The model under review builds one solid part; all positions refer to its coordinate system, in mm. Face numbers are marked on the shaded views. A direction names the side the tool comes from. Round coordinates to 2 decimals unless told otherwise and drop trailing zeros. Loops run counter-clockwise (first coordinate to the right, second up) from the corner with the lowest first, then second, coordinate; pieces in that order, holes last. Notation, with made-up numbers: (-13, -18.5) - (-9, -18.5) arc R24 cw to (-9, 19.5) - close; hole circle Ø11 at (-27, -18.5). An arc over 180 degrees is marked (long way). Answer as CSV lines item,"result".
Autodesk Fusion 360 part; units mm, degrees
sketch "Sketch1" plane through (0, 0, 0) normal (0, 0, 1) x (1, 0, 0)
  line L0 (67.5, 27.5) -> (-67.5, 27.5)
  line L1 (-67.5, 27.5) -> (-67.5, -27.5)
  line L2 (-67.5, -27.5) -> (67.5, -27.5)
  line L3 (67.5, -27.5) -> (67.5, 27.5)
  line L4 (67.5, 27.5) -> (-67.5, -27.5) construction
  line L5 (-67.5, 27.5) -> (67.5, -27.5) construction
  dimension "d1" = 55
  dimension "d2" = 135
extrude "Extrude1" add sketch "Sketch1" along normal blind 6 makes body 1
sketch "Sketch3" plane through (0, 0, 0) normal (0, 0, -1) x (-1, 0, 0)
  line L0 (-67.5, 27.5) -> (-67.5, -27.5)
  line L1 (-67.5, -27.5) -> (67.5, -27.5)
  line L2 (67.5, -27.5) -> (67.5, 27.5)
  line L3 (67.5, 27.5) -> (-67.5, 27.5)
  line L4 (-67.5, -7) -> (67.5, -7)
  line L5 (67.5, -7) -> (67.5, 27.5)
  line L6 (67.5, 27.5) -> (-67.5, 27.5)
  line L7 (-67.5, 27.5) -> (-67.5, -7)
  line L8 (-67.5, -7) -> (67.5, 27.5) construction
  line L9 (67.5, -7) -> (-67.5, 27.5) construction
  point P0 (0, 10.25)
  dimension "d14" = 34.5
  dimension "d30" = 20.5
extrude "Extrude2" add sketch "Sketch3" along normal blind 6 contours L0 L2 L3 L4 L5 L6 L7 bodies 1
sketch "Sketch4" plane through (0, 0, -6) normal (0, 0, -1) x (-1, 0, 0)
  line L0 (-67.5, 27.5) -> (-67.5, -7)
  line L1 (-67.5, -7) -> (67.5, -7)
  line L2 (67.5, -7) -> (67.5, 27.5)
  line L3 (67.5, 27.5) -> (-67.5, 27.5)
  line L4 (-67.5, 4.75) -> (67.5, 4.75) construction
  point P0 (54.75, 4.75)
  point P1 (-31.75, 4.75)
  dimension "d19" = 12.75
  dimension "d20" = 86.5
  dimension "d31" = 11.75
hole "Hole2" at (31.75, 4.75, -6) at (-54.75, 4.75, -6) direction (0, 0, 1) diameter 3.5 end through all bodies 1 1
sketch "Sketch5" plane through (0, 0, 6) normal (0, 0, 1) x (1, 0, 0)
  circle A0 centre (31.75, 4.75) radius 1.75
  circle A1 centre (-54.75, 4.75) radius 1.75
  line L0 (67.5, -27.5) -> (67.5, 27.5)
  line L1 (67.5, 27.5) -> (-67.5, 27.5)
  line L2 (-67.5, 27.5) -> (-67.5, -27.5)
  line L3 (-67.5, -27.5) -> (67.5, -27.5)
  line L4 (-51.65, 6.5398) -> (-54.75, 8.3296)
  line L5 (-54.75, 8.3296) -> (-57.85, 6.5398)
  line L6 (-57.85, 6.5398) -> (-57.85, 2.9602)
  line L7 (-57.85, 2.9602) -> (-54.75, 1.1704)
  line L8 (-54.75, 1.1704) -> (-51.65, 2.9602)
  line L9 (-51.65, 2.9602) -> (-51.65, 6.5398)
  line L10 (34.85, 2.9602) -> (34.85, 6.5398)
  line L11 (34.85, 6.5398) -> (31.75, 8.3296)
  line L12 (31.75, 8.3296) -> (28.65, 6.5398)
  line L13 (28.65, 6.5398) -> (28.65, 2.9602)
  line L14 (28.65, 2.9602) -> (31.75, 1.1704)
  line L15 (31.75, 1.1704) -> (34.85, 2.9602)
  point P0 (-54.75, 4.75)
  point P1 (31.75, 4.75)
  dimension "d24" = 6.2
  dimension "d25" = 6.2
extrude "Extrude3" cut sketch "Sketch5" against normal blind 6 contours L4 L5 L6 L7 L8 L9 | L10 L11 L12 L13 L14 L15 bodies 1
sketch "Sketch6" plane through (0, 0, -6) normal (0, 0, -1) x (-1, 0, 0)
  circle A0 centre (-31.75, 4.75) radius 1.75
  circle A1 centre (54.75, 4.75) radius 1.75
  line L0 (-67.5, 27.5) -> (-67.5, -7)
  line L1 (-67.5, -7) -> (67.5, -7)
  line L2 (67.5, -7) -> (67.5, 27.5)
  line L3 (67.5, 27.5) -> (-67.5, 27.5)
  line L4 (59.5, -7) -> (-36.5, -7) construction
  line L5 (-36.5, -7) -> (-36.5, 28) construction
  line L6 (-36.5, 28) -> (59.5, 28) construction
  line L7 (59.5, 28) -> (59.5, -7) construction
  line L8 (59.5, -7) -> (-36.5, 28) construction
  line L9 (-36.5, -7) -> (59.5, 28) construction
  line L10 (11.5, 50.5144) -> (11.5, -41.0982) construction
  line L11 (-52, 27.5) -> (-52, -7) construction
  line L12 (-36.5, 10.25) -> (-67.5, 10.25) construction
  point P0 (11.5, 10.5)
  point P1 (-52, 10.25)
  dimension "d28" = 35
  dimension "d29" = 96
hole "Hole3" at (52, 10.25, -6) direction (0, 0, 1) diameter 5.5 end through all bodies 1 1
fillet "Fillet1" radius 5 2 edges at (67.5, -27.5, 3) (-67.5, -27.5, 3) on bodies 1
fillet "Fillet1" radius 5 1 edges at (-67.5, 27.5, 0) on bodies 1
fillet "Fillet3" radius 15 1 edges at (67.5, 27.5, 0) on bodies 1
ref_plane "WorkPlane1" through (0, -27.5, 3) normal (0, -1, 0) x (1, 0, 0)
mirror "Mirror1" about plane through (0, -27.5, 3) normal (0, -1, 0) of bodies 1 makes body 2
sketch "Sketch8" plane through (0, 0, 6) normal (0, 0, 1) x (1, 0, 0)
  arc A0 (52.5, -82.5) -> (67.5, -67.5) centre (52.5, -67.5) ccw
  line L0 (67.5, -67.5) -> (67.5, -32.5)
  arc A1 (67.5, -32.5) -> (62.5, -27.5) centre (62.5, -32.5) ccw
  line L1 (62.5, -27.5) -> (-62.5, -27.5)
  arc A2 (-62.5, -27.5) -> (-67.5, -32.5) centre (-62.5, -32.5) ccw
  line L2 (-67.5, -32.5) -> (-67.5, -77.5)
  arc A3 (-67.5, -77.5) -> (-62.5, -82.5) centre (-62.5, -77.5) ccw
  line L3 (-62.5, -82.5) -> (52.5, -82.5)
  circle A4 centre (52, -65.25) radius 2.75
  line L4 (-51.65, -61.5398) -> (-54.75, -63.3296)
  line L5 (-54.75, -63.3296) -> (-57.85, -61.5398)
  line L6 (-57.85, -61.5398) -> (-57.85, -57.9602)
  line L7 (-57.85, -57.9602) -> (-54.75, -56.1704)
  line L8 (-54.75, -56.1704) -> (-51.65, -57.9602)
  line L9 (-51.65, -57.9602) -> (-51.65, -61.5398)
  line L10 (34.85, -57.9602) -> (34.85, -61.5398)
  line L11 (34.85, -61.5398) -> (31.75, -63.3296)
  line L12 (31.75, -63.3296) -> (28.65, -61.5398)
  line L13 (28.65, -61.5398) -> (28.65, -57.9602)
  line L14 (28.65, -57.9602) -> (31.75, -56.1704)
  line L15 (31.75, -56.1704) -> (34.85, -57.9602)
  arc A5 (-62.5, -27.5) -> (-67.5, -32.5) centre (-62.5, -32.5) ccw
  line L16 (-62.5, -27.5) -> (62.5, -27.5)
  arc A6 (67.5, -32.5) -> (62.5, -27.5) centre (62.5, -32.5) ccw
  line L17 (67.5, -32.5) -> (67.5, -48)
  line L18 (67.5, -48) -> (-67.5, -48)
  line L19 (-67.5, -48) -> (-67.5, -32.5)
  point P0 (-44.5, -41)
  point P1 (37, -41)
  dimension "d58" = 7
  dimension "d60" = 7
  dimension "d61" = 30.5
  dimension "d67" = 81.5
hole "Hole4" at (-44.5, -41, 6) at (37, -41, 6) direction (0, 0, -1) diameter 3.5 end through all counterbore diameter 6.5 counterbore depth 3.25 bodies 2 2
fillet "Fillet4" radius 1 1 edges at (0, -48, -6) on bodies 2
fillet "Fillet5" radius 0.5 14 edges at (-67.5, -40.25, 0) (-66.0355, -28.9645, 0) (0, -27.5, 0) (66.0355, -28.9645, 0) (67.5, -40.25, 0) (-67.5, -48, -2.5) (-67.5, -48.2929, -5.7071) (-67.5, -63.25, -6) (-66.0355, -81.0355, -6) (-5, -82.5, -6) (63.1066, -78.1066, -6) (67.5, -58.25, -6) (67.5, -48.2929, -5.7071) (67.5, -48, -2.5) on bodies 2
sketch "Sketch9" plane through (0, 0, -6) normal (0, 0, -1) x (-1, 0, 0)
  circle A0 centre (-52, -65.25) radius 2.75
  circle A1 centre (-31.75, -59.75) radius 1.75
  circle A2 centre (54.75, -59.75) radius 1.75
  line L0 (-67, -49) -> (-67, -67.5)
  arc A3 (-67, -67.5) -> (-52.5, -82) centre (-52.5, -67.5) ccw
  line L1 (-52.5, -82) -> (62.5, -82)
  arc A4 (62.5, -82) -> (67, -77.5) centre (62.5, -77.5) ccw
  line L2 (67, -77.5) -> (67, -49)
  line L3 (67, -49) -> (-67, -49)
  line L4 (48.25, -77.5) -> (-25.25, -77.5)
  line L5 (-25.25, -77.5) -> (-25.25, -53)
  line L6 (-25.25, -53) -> (48.25, -53)
  line L7 (48.25, -53) -> (48.25, -77.5)
  line L8 (48.25, -77.5) -> (-25.25, -53) construction
  line L9 (-25.25, -77.5) -> (48.25, -53) construction
  line L10 (67, -48) -> (-67, -48)
  line L11 (-52.5, -82.5) -> (62.5, -82.5)
  point P0 (11.5, -65.25)
  dimension "d68" = 5
  dimension "d69" = 5
  dimension "d71" = 6.5
  dimension "d82" = 6.5
extrude "Extrude4" cut sketch "Sketch9" against normal through all contours L4 L5 L6 L7 bodies 2
fillet "Fillet6" radius 5 4 edges at (25.25, -53, 0) (25.25, -77.5, 0) (-48.25, -77.5, 0) (-48.25, -53, 0) on bodies 2
sketch "Sketch10" plane through (0, 0, 0) normal (0, 0, -1) x (-1, 0, 0)
  line L0 (-67, -32.5) -> (-67, -48)
  line L1 (-67, -48) -> (67, -48)
  line L2 (67, -48) -> (67, -32.5)
  arc A0 (67, -32.5) -> (62.5, -28) centre (62.5, -32.5) ccw
  line L3 (62.5, -28) -> (-62.5, -28)
  arc A1 (-62.5, -28) -> (-67, -32.5) centre (-62.5, -32.5) ccw
  circle A2 centre (44.5, -41) radius 1.75
  circle A3 centre (-37, -41) radius 1.75
  line L4 (38, -43) -> (-30.5, -43)
  line L5 (-30.5, -43) -> (-30.5, -32.5)
  line L6 (-30.5, -32.5) -> (38, -32.5)
  line L7 (38, -32.5) -> (38, -43)
  line L8 (38, -43) -> (-30.5, -32.5) construction
  line L9 (-30.5, -43) -> (38, -32.5) construction
  line L10 (62.5, -27.5) -> (-62.5, -27.5)
  point P0 (3.75, -37.75)
  dimension "d75" = 5
  dimension "d76" = 5
  dimension "d77" = 6.5
  dimension "d78" = 6.5
extrude "Extrude5" cut sketch "Sketch10" against normal through all contours L4 L5 L6 L7 bodies 2
fillet "Fillet7" radius 5 4 edges at (-38, -43, 3) (-38, -32.5, 3) (30.5, -32.5, 3) (30.5, -43, 3) on bodies 2
hidden bodies 1
equation "d19 = 15 mm - 2.25 mm"
equation "d20 = 82 mm + 4.5 mm"
equation "d25 = d24"
equation "d31 = 9.5 mm + 2.25 mm"
equation "d69 = d68"
equation "d71 = d82"
equation "d76 = d75"
equation "d78 = d77"
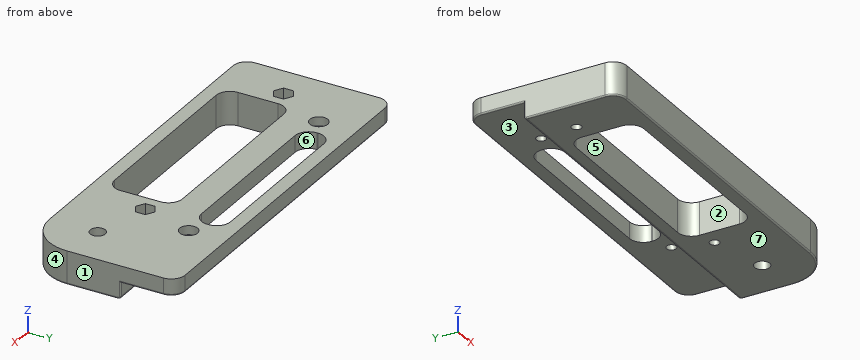
1. Clearance check with flat-ended pins moving along their axes: pin 1 (6 mm diameter, centred on x = -44.5, y = -41, fed in from -Z); pin 2 (4 mm diameter, centred on x = 37, y = -41, fed in from +Z); pin 3 (4.5 mm diameter, centred on x = 52, y = -65.25, fed in from +Z); pin 4 (4 mm diameter, centred on x = 31.75, y = -59.75, fed in from +Z). State where each tip first meets the part, or that it passes through.
Numbers:
pin 1,"stops at z = 0"
pin 2,"stops at z = 2.75"
pin 3,"passes through"
pin 4,"stops at z = 0"
2. Take a section at D-D (x = -44.5). State the section outline as (y, z) points, plus the area to 3 significant figures.
Numbers:
outline,"(-82.5, -5.5) arc R0.5 ccw to (-82, -6) - (-77.34, -6) - (-77.34, 6) - (-82.5, 6) - close; (-53.16, -6) - (-49, -6) arc R1 ccw to (-48, -5) - (-48, 0) - (-42.75, 0) - (-42.75, 2.75) - (-44.25, 2.75) - (-44.25, 6) - (-53.16, 6) - close; (-39.25, 0) - (-28, 0) arc R0.5 ccw to (-27.5, 0.5) - (-27.5, 6) - (-37.75, 6) - (-37.75, 2.75) - (-39.25, 2.75) - close"
area,"216 mm²"
3. Wall thickness on probe 1 along Y at (x, z) = (-15.5, 1.5); probe 2 along X at (y, z) = (-59.75, -4.4); probe 3 along X at (y, z) = (-59, 1.25): over which ranges is each line inside the solid? List them lowest first.
Numbers:
probe 1,"y = -82.5 to -77.5, -53 to -43, -32.5 to -27.5"
probe 2,"x = -67.5 to -56.5, -53 to -48.25, 25.25 to 30, 33.5 to 67.5"
probe 3,"x = -67.5 to -57.85, -51.65 to -48.25, 25.25 to 28.65, 34.85 to 67.5"
4. Take a section at C-C (x = 37). State the section outline as (y, z) points.
Numbers:
outline,"(-82.5, -5.5) arc R0.5 ccw to (-82, -6) - (-49, -6) arc R1 ccw to (-48, -5) - (-48, 0) - (-42.75, 0) - (-42.75, 2.75) - (-44.25, 2.75) - (-44.25, 6) - (-82.5, 6) - close; (-39.25, 0) - (-28, 0) arc R0.5 ccw to (-27.5, 0.5) - (-27.5, 6) - (-37.75, 6) - (-37.75, 2.75) - (-39.25, 2.75) - close"
5. Take a section at B-B (z = -3.75). State the section outline as (x, y) points, plus the area to 3 significant figures.
Numbers:
outline,"(-67.5, -77.5) arc R5 ccw to (-62.5, -82.5) - (52.5, -82.5) arc R15 ccw to (67.5, -67.5) - (67.5, -48.5) arc R0.5 ccw to (67, -48) - (-67, -48) arc R0.5 ccw to (-67.5, -48.5) - close; hole circle Ø3.5 at (-54.75, -59.75); hole (-48.25, -72.5) arc R5 ccw to (-43.25, -77.5) - (20.25, -77.5) arc R5 ccw to (25.25, -72.5) - (25.25, -58) arc R5 ccw to (20.25, -53) - (-43.25, -53) arc R5 ccw to (-48.25, -58) - close; hole circle Ø3.5 at (31.75, -59.75); hole circle Ø5.5 at (52, -65.25)"
area,"2,780 mm²"
6. Take a section at A-A (x = -15). State the section outline as (y, z) points.
Numbers:
outline,"(-82.5, -5.5) arc R0.5 ccw to (-82, -6) - (-77.5, -6) - (-77.5, 6) - (-82.5, 6) - close; (-53, -6) - (-49, -6) arc R1 ccw to (-48, -5) - (-48, 0) - (-43, 0) - (-43, 6) - (-53, 6) - close; (-32.5, 0) - (-28, 0) arc R0.5 ccw to (-27.5, 0.5) - (-27.5, 6) - (-32.5, 6) - close"
7. Tool access review of the marked faces 1, 2 and 3: name each direction out of +Z, -Z, +X, -X, +Y, -Y from which nothing blocks a thin tool from reaching the whole face with its end or side.
Numbers:
face 1,"+Z, -Z, +X, +Y, -Y"
face 2,"+Z, -Z"
face 3,"-Z, +X, -X, +Y"
8. Draft analysis for pull direction X (two halves, no side actions). For the marked faces 4, 5, 6 and 7, state which applies: +X half, -X half, draft (parallel to the pull), parting line (faces both ways), or undercut.
Numbers:
face 4,"+X half"
face 5,"undercut"
face 6,"undercut"
face 7,"draft"
